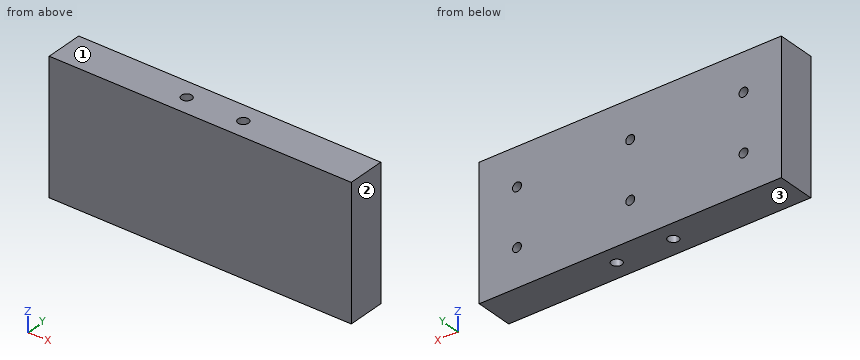
from build123d import *

# Parameters (mm, degrees)
SKETCH1_W                 = 44.45
SKETCH1_H                 = 12.7
BOSS_EXTRUDE1_DEPTH       = 50.8
M3_10_THREADED_HOLE_D     = 3
M3_10_THREADED_HOLE_DEPTH = 6.35
M3_10_THREADED_HOLE_TIP   = 0.901290929
F_6_32_THREADED_HOLE_D    = 3.51028


with BuildPart() as part:
    # Sketch1 → Boss-Extrude1 (new, symmetric)
    with BuildSketch(Plane(origin=(0, 0, 0), x_dir=(0, 0, -1), z_dir=(1, 0, 0))):
        Rectangle(SKETCH1_W, SKETCH1_H)
    extrude(amount=BOSS_EXTRUDE1_DEPTH, both=True)

    # M3-10 Threaded Hole
    with Locations(Plane(origin=(0, 6.35, 0), x_dir=(1, 0, 0), z_dir=(0, 1, 0))):
        with Locations((-38.1, -9.525), (0, -9.525), (38.1, -9.525), (-38.1, 9.525), (0, 9.525), (38.1, 9.525)):
            Hole(M3_10_THREADED_HOLE_D / 2, depth=M3_10_THREADED_HOLE_DEPTH)
            with Locations((0, 0, -(M3_10_THREADED_HOLE_DEPTH + M3_10_THREADED_HOLE_TIP / 2))):  # 118° drill point
                Cone(0, M3_10_THREADED_HOLE_D / 2, M3_10_THREADED_HOLE_TIP, mode=Mode.SUBTRACT)

    # #6-32 Threaded Hole (through all)
    with Locations(Plane.XY.offset(22.225)):
        with Locations((-9.525, 0), (9.525, 0)):
            Hole(F_6_32_THREADED_HOLE_D / 2)


solid = part.part
Check sheet for the modelled part. Datum: model origin and axes. Units: mm. Face numbers are marked on the shaded views. Coordinates: 2 decimals unless noted, no trailing zeros. Write each loop counter-clockwise with the first axis right and the second up, starting at its lowest first coordinate (ties: lowest second). Pieces come first, ordered by that corner, then holes.
Item 1: Scan lines: probe 1 along Z at (x, y) = (38.1, 3) (3 decimals); probe 2 along X at (y, z) = (-0.25, 1); probe 3 along X at (y, z) = (1.5, 16.5). Record each from-to range of solid material in increasing order.
Numbers:
probe 1: z = -22.225 to -11.025, -8.025 to 8.025, 11.025 to 22.225
probe 2: x = -50.8 to -11.26, -7.79 to 7.79, 11.26 to 50.8
probe 3: x = -50.8 to -10.44, -8.61 to 8.61, 10.44 to 50.8
Item 2: Mould release check, pull along Z, two halves, no side actions. Record for the marked faces 1, 2 and 3: released by +Z, released by -Z, zero draft, split by the parting line, or undercut.
Numbers:
face 1: released by +Z
face 2: zero draft
face 3: released by -Z
Item 3: Cross-section at B-B on z = 2. Record the boundary of the cut face in (x, y) (3 decimals), then the cut area to 3 significant figures.
Numbers:
outline: (-50.8, -6.35) - (50.8, -6.35) - (50.8, 6.35) - (-50.8, 6.35) - close; hole circle Ø3.51 at (-9.525, 0); hole circle Ø3.51 at (9.525, 0)
area: 1,270 mm2
Item 4: Depth check by flat-ended pin: pin 1 Ø2.5 at (x, z) = (0, 9.525) entering from +Y. Enter the tip coordinate at first touch or a pass-through.
Numbers:
pin 1: stops at y = -0.15
Item 5: Cross-section at A-A on x = 9. Record the boundary of the cut face in (y, z) (3 decimals).
Numbers:
outline: (-6.35, -22.225) - (-1.675, -22.225) - (-1.675, 22.225) - (-6.35, 22.225) - close; (1.675, -22.225) - (6.35, -22.225) - (6.35, 22.225) - (1.675, 22.225) - close
